from build123d import *

# Parameters (mm, degrees)
CIRCLE_DEPTH       = 5
SKETCH2_W          = 100
SKETCH2_H          = 100
SQUARE_DEPTH       = 5
SKETCH3_R          = 2.5
HOLES_DEPTH        = 5
CUT_EXTRUDE3_DEPTH = 5


with BuildPart() as part:
    # Sketch1 → circle (new body)
    with BuildSketch(Plane.XY):
        with BuildLine():
            Line((-31.416556145, -67), (31.416556145, -67))
            ThreePointArc((31.416556145, -67), (0, 74), (-31.416556145, -67))
        make_face()
    extrude(amount=CIRCLE_DEPTH)

    # Sketch2 → square (cut)
    with BuildSketch(Plane.XY.offset(5)):
        Rectangle(SKETCH2_W, SKETCH2_H)
    extrude(amount=-SQUARE_DEPTH, mode=Mode.SUBTRACT)

    # Sketch3 → holes (cut)
    with BuildSketch(Plane.XY.offset(5)):
        with Locations((0, 60)):
            Circle(SKETCH3_R)
        with Locations((0, -60)):
            Circle(SKETCH3_R)
    extrude(amount=-HOLES_DEPTH, mode=Mode.SUBTRACT)

    # Sketch4 → Cut-Extrude3 (cut)
    with BuildSketch(Plane.XY.offset(5)):
        Polygon((-50, 0), (-50, -8.3), (-57.55, -8.3), (-60.903744176, -10), (-67.80719259, -6.5), (-67.80719259, 6.5), (-60.903744176, 10), (-57.55, 8.3), (-50, 8.3), align=None)
        Polygon((57.55, 8.3), (50, 8.3), (50, 0), (50, -8.3), (57.55, -8.3), (60.903744176, -10), (67.80719259, -6.5), (67.80719259, 6.5), (60.903744176, 10), align=None)
    extrude(amount=-CUT_EXTRUDE3_DEPTH, mode=Mode.SUBTRACT)


solid = part.part
Source: CAD feature listing. Evaluate the final solid. Frame: model axes, mm. A direction names the side the tool comes from. Round coordinates to 2 decimals unless told otherwise and drop trailing zeros. Write each loop counter-clockwise with the first axis right and the second up, starting at its lowest first coordinate (ties: lowest second). Pieces come first, ordered by that corner, then holes. Notation, with made-up numbers: M -4,84.5 L 25,84.5 A6 cw 25,94.5 Z; hole C 62.5,5 d2. An arc over 180 degrees is marked long. One line per item, written item: value. Start each with the question number.
Item 1: Set-up query: faces 1 (the flat face through (0, -67, 2)), 2 (the flat face through (-67.807, 0, 3)). Return all of +Z, -Z, +X, -X, +Y, -Y with unobstructed straight access to the full face (end or side cutting, diameter ignored); none if empty.
Item 2: Section query D-D (x = -64.5). Return the cut outline in (y, z), plus the area to 3 significant figures.
Item 3: Pin query (flat end, axial travel): pin 1 (2.5 mm diameter, centred on x = 53.5, z = 3.5, fed in from +Y); pin 2 (1.5 mm diameter, centred on x = -55, z = 2, fed in from +Y); pin 3 (1.5 mm diameter, centred on y = 27, z = 3, fed in from +X). Return the tip coordinate at first contact, or that it passes through.
Item 4: Section query B-B (y = 0). Return the cut outline in (x, z).
Item 5: Ray query, L1, parallel to Y at x = 0, z = 3.4; L2, parallel to Y at x = -24, z = 1.5; L3, parallel to Y at x = -5, z = 1.95. Return the intervals inside material, ascending. Write a range as from..to.
Item 6: Section query A-A (z = 3.25). Return the cut outline in (x, y).
Item 7: Section query C-C (x = 0). Return the cut outline in (y, z).
Item 8: Mould query, pull axis Y, two halves, no side actions, for faces 3 (the flat face through (0, 51, 0)), 4 (the flat face through (54, 8.3, 3)), 5 (the cylindrical face through (2.8, 73.947, 2.465)), 6 (the cylindrical face through (1.34, -57.89, 2.54)). Classes: pulls with the +Y half, pulls with the -Y half, needs draft (parallel to the pull), parting line crosses it, or undercut.
Result set:
1. face 1: +Z, -Z, +X, -X, -Y
1. face 2: +Z, -Z
2. outline: M -36.27,0 L -8.18,0 L -8.18,5 L -36.27,5 Z; M 8.18,0 L 36.27,0 L 36.27,5 L 8.18,5 Z
2. area: 281 mm²
3. pin 1: stops at y = 52.4
3. pin 2: stops at y = 50.33
3. pin 3: stops at x = 69.19
4. outline: M -74,0 L -67.81,0 L -67.81,5 L -74,5 Z; M 67.81,0 L 74,0 L 74,5 L 67.81,5 Z
5. L1: y = -67..-62.5, -57.5..-50, 50..57.5, 62.5..74
5. L2: y = -67..-50, 50..70
5. L3: y = -67..-50, 50..73.83
6. outline: M -31.42,-67 L 31.42,-67 A74 ccw long Z; hole M -67.81,-6.5 L -60.9,-10 L -57.55,-8.3 L -50,-8.3 L -50,-50 L 50,-50 L 50,-8.3 L 57.55,-8.3 L 60.9,-10 L 67.81,-6.5 L 67.81,6.5 L 60.9,10 L 57.55,8.3 L 50,8.3 L 50,50 L -50,50 L -50,8.3 L -57.55,8.3 L -60.9,10 L -67.81,6.5 Z; hole C 0,-60 d5; hole C 0,60 d5
7. outline: M -67,0 L -62.5,0 L -62.5,5 L -67,5 Z; M -57.5,0 L -50,0 L -50,5 L -57.5,5 Z; M 50,0 L 57.5,0 L 57.5,5 L 50,5 Z; M 62.5,0 L 74,0 L 74,5 L 62.5,5 Z
8. face 3: needs draft
8. face 4: undercut
8. face 5: parting line crosses it
8. face 6: undercut
